The model under review builds one solid part; all positions refer to its coordinate system, in mm. A direction names the side the tool comes from. Round coordinates to 2 decimals unless told otherwise and drop trailing zeros. Order: outer loops, then holes, each group sorted by start corner. A loop starts at its lowest first (then second) coordinate and runs counter-clockwise, first axis right, second up. Notation, with made-up numbers: M 69,64 L 98,64 A22 ccw 98,88 Z; hole C -10,26 d1. An arc over 180 degrees is marked long. Answer as a JSON object with one key per item and string values. Group by question number.
1. To check wall thickness, follow probe 1 along Y at (x, z) = (0, 30); probe 2 along X at (y, z) = (3.75, 18.5); probe 3 along X at (y, z) = (-1, 36). State the ranges of each line that lie inside material, in increasing order. Write a range as [from, to].
2. Mouldability with a two-part tool opening along Y and no side actions: class faces 1 (the face through (-4, -2, 20)), 2 (the face through (5, 3, 20)), 3 (the face through (3, -5, 20)) as released by +Y, released by -Y, zero draft, split by the parting line, or undercut.
3. Add section A-A on y = 0. State the section outline as (x, z) points.
4. Clearance check with a flat-ended pin moving along its axis: P1, Ø1.6, axis at x = 0, z = 26.5, coming from the +Y side. State where the tip first meets the part, or that it passes through.
5. Machinability: for faces 4 (the face through (0, -2, 20)), 5 (the face through (2, 0, 20)), 6 (the face through (-1.995, 2.835, 19.72)), 7 (the face through (-2, 0, 20)), which of the approach directions +Z, -Z, +X, -X, +Y, -Y give a long, thin tool a straight path to every point of the face, cutting with its end or side? Answer none if there is none.
```python
from build123d import *

# Parameters (mm, degrees)
SKETCH1_R           = 1.25
BOSS_EXTRUDE1_DEPTH = 40


with BuildPart() as part:
    # Sketch1 → Boss-Extrude1 (new body)
    with BuildSketch(Plane.XY):
        with BuildLine():
            Line((-4.8, 5), (-1.7, 5))
            ThreePointArc((-1.7, 5), (-1.558578644, 4.941421356), (-1.5, 4.8))
            Line((-1.5, 4.8), (-1.5, 4.2))
            ThreePointArc((-1.5, 4.2), (-1.558578644, 4.058578644), (-1.7, 4))
            Line((-1.7, 4), (-2.834011701, 4))
            ThreePointArc((-2.834011701, 4), (-3.021950225, 3.868404029), (-2.962569223, 3.646791111))
            Line((-2.962569223, 3.646791111), (-1, 2))
            Line((-1, 2), (1, 2))
            Line((1, 2), (2.962569223, 3.646791111))
            ThreePointArc((2.962569223, 3.646791111), (3.021950225, 3.868404029), (2.834011701, 4))
            Line((2.834011701, 4), (1.7, 4))
            ThreePointArc((1.7, 4), (1.558578644, 4.058578644), (1.5, 4.2))
            Line((1.5, 4.2), (1.5, 4.8))
            ThreePointArc((1.5, 4.8), (1.558578644, 4.941421356), (1.7, 5))
            Line((1.7, 5), (4.8, 5))
            ThreePointArc((4.8, 5), (4.941421356, 4.941421356), (5, 4.8))
            Line((5, 4.8), (5, 1.7))
            ThreePointArc((5, 1.7), (4.941421356, 1.558578644), (4.8, 1.5))
            Line((4.8, 1.5), (4.2, 1.5))
            ThreePointArc((4.2, 1.5), (4.058578644, 1.558578644), (4, 1.7))
            Line((4, 1.7), (4, 2.834011701))
            ThreePointArc((4, 2.834011701), (3.868404029, 3.021950225), (3.646791111, 2.962569223))
            Line((3.646791111, 2.962569223), (2, 1))
            Line((2, 1), (2, -1))
            Line((2, -1), (3.646791111, -2.962569223))
            ThreePointArc((3.646791111, -2.962569223), (3.868404029, -3.021950225), (4, -2.834011701))
            Line((4, -2.834011701), (4, -1.7))
            ThreePointArc((4, -1.7), (4.058578644, -1.558578644), (4.2, -1.5))
            Line((4.2, -1.5), (4.8, -1.5))
            ThreePointArc((4.8, -1.5), (4.941421356, -1.558578644), (5, -1.7))
            Line((5, -1.7), (5, -4.8))
            ThreePointArc((5, -4.8), (4.941421356, -4.941421356), (4.8, -5))
            Line((4.8, -5), (1.7, -5))
            ThreePointArc((1.7, -5), (1.558578644, -4.941421356), (1.5, -4.8))
            Line((1.5, -4.8), (1.5, -4.2))
            ThreePointArc((1.5, -4.2), (1.558578644, -4.058578644), (1.7, -4))
            Line((1.7, -4), (2.834011701, -4))
            ThreePointArc((2.834011701, -4), (3.021950225, -3.868404029), (2.962569223, -3.646791111))
            Line((2.962569223, -3.646791111), (1, -2))
            Line((1, -2), (-1, -2))
            Line((-1, -2), (-2.962569223, -3.646791111))
            ThreePointArc((-2.962569223, -3.646791111), (-3.021950225, -3.868404029), (-2.834011701, -4))
            Line((-2.834011701, -4), (-1.7, -4))
            ThreePointArc((-1.7, -4), (-1.558578644, -4.058578644), (-1.5, -4.2))
            Line((-1.5, -4.2), (-1.5, -4.8))
            ThreePointArc((-1.5, -4.8), (-1.558578644, -4.941421356), (-1.7, -5))
            Line((-1.7, -5), (-4.8, -5))
            ThreePointArc((-4.8, -5), (-4.941421356, -4.941421356), (-5, -4.8))
            Line((-5, -4.8), (-5, -1.7))
            ThreePointArc((-5, -1.7), (-4.941421356, -1.558578644), (-4.8, -1.5))
            Line((-4.8, -1.5), (-4.2, -1.5))
            ThreePointArc((-4.2, -1.5), (-4.058578644, -1.558578644), (-4, -1.7))
            Line((-4, -1.7), (-4, -2.834011701))
            ThreePointArc((-4, -2.834011701), (-3.868404029, -3.021950225), (-3.646791111, -2.962569223))
            Line((-3.646791111, -2.962569223), (-2, -1))
            Line((-2, -1), (-2, 1))
            Line((-2, 1), (-3.646791111, 2.962569223))
            ThreePointArc((-3.646791111, 2.962569223), (-3.868404029, 3.021950225), (-4, 2.834011701))
            Line((-4, 2.834011701), (-4, 1.7))
            ThreePointArc((-4, 1.7), (-4.058578644, 1.558578644), (-4.2, 1.5))
            Line((-4.2, 1.5), (-4.8, 1.5))
            ThreePointArc((-4.8, 1.5), (-4.941421356, 1.558578644), (-5, 1.7))
            Line((-5, 1.7), (-5, 4.8))
            ThreePointArc((-5, 4.8), (-4.941421356, 4.941421356), (-4.8, 5))
        make_face()
        Circle(SKETCH1_R, mode=Mode.SUBTRACT)
    extrude(amount=BOSS_EXTRUDE1_DEPTH)


solid = part.part
```
Recorded:
{
 "1": {"probe 1": "y = [-2, -1.25], [1.25, 2]", "probe 2": "x = [-5, -3.03], [3.03, 5]", "probe 3": "x = [-2, -0.75], [0.75, 2]"},
 "2": {"face 1": "undercut", "face 2": "zero draft", "face 3": "released by -Y"},
 "3": {"outline": "M -2,0 L -1.25,0 L -1.25,40 L -2,40 Z; M 1.25,0 L 2,0 L 2,40 L 1.25,40 Z"},
 "4": {"P1": "stops at y = 2"},
 "5": {"face 4": "+Z, -Z, -Y", "face 5": "+Z, -Z, +X", "face 6": "+Z, -Z", "face 7": "+Z, -Z, -X"}
}
